from build123d import *

# Parameters (mm, degrees)
CROQUIS1_W              = 31.5
CROQUIS1_H              = 126
SALIENTE_EXTRUIR1_DEPTH = 4
CROQUIS3_R              = 2
CORTAR_EXTRUIR2_DEPTH   = 5
CROQUIS8_R              = 2.55
CORTAR_EXTRUIR3_DEPTH   = 5
CROQUIS11_R             = 1.575
CORTAR_EXTRUIR8_DEPTH   = 5
CROQUIS15_R             = 1.575
CORTAR_EXTRUIR11_DEPTH  = 5
CHAFL_N2_SIZE           = 3
CROQUIS19_R             = 3.5
CORTAR_EXTRUIR13_DEPTH  = 1.9
CROQUIS20_R             = 3.05
CORTAR_EXTRUIR14_DEPTH  = 2
CROQUIS24_W             = 31.5
CROQUIS24_H             = 3.76
SALIENTE_EXTRUIR3_DEPTH = 4
CROQUIS25_R             = 2.025
CORTAR_EXTRUIR15_DEPTH  = 5


with BuildPart() as part:
    # Croquis1 → Saliente-Extruir1 (new body)
    with BuildSketch(Plane(origin=(0, 0, 0), x_dir=(0, 0, -1), z_dir=(1, 0, 0))):
        Rectangle(CROQUIS1_W, CROQUIS1_H)
    extrude(amount=SALIENTE_EXTRUIR1_DEPTH)

    # Croquis3 → Cortar-Extruir2 (cut, through all)
    with BuildSketch(Plane(origin=(4, 0, 0), x_dir=(0, 0, -1), z_dir=(1, 0, 0))):
        with Locations((-10, 10.1)):
            Circle(CROQUIS3_R)
        with Locations((10, 10.1)):
            Circle(CROQUIS3_R)
        with Locations((-10, -9.9)):
            Circle(CROQUIS3_R)
        with Locations((10, -9.9)):
            Circle(CROQUIS3_R)
    extrude(amount=-CORTAR_EXTRUIR2_DEPTH, mode=Mode.SUBTRACT)

    # Croquis8 → Cortar-Extruir3 (cut, through all)
    with BuildSketch(Plane.ZY):
        with Locations((0, 45.75)):
            Circle(CROQUIS8_R)
    extrude(amount=-CORTAR_EXTRUIR3_DEPTH, mode=Mode.SUBTRACT)

    # Croquis11 → Cortar-Extruir8 (cut, through all)
    with BuildSketch(Plane(origin=(4, 0, 0), x_dir=(0, 0, -1), z_dir=(1, 0, 0))):
        with Locations((2.75, 34.75)):
            Circle(CROQUIS11_R)
        with Locations((2.75, 24.75)):
            Circle(CROQUIS11_R)
    extrude(amount=-CORTAR_EXTRUIR8_DEPTH, mode=Mode.SUBTRACT)

    # Croquis15 → Cortar-Extruir11 (cut, through all)
    with BuildSketch(Plane(origin=(4, 0, 0), x_dir=(0, 0, -1), z_dir=(1, 0, 0))):
        with Locations((-11.15, 57.45)):
            Circle(CROQUIS15_R)
        with Locations((11.15, 57.45)):
            Circle(CROQUIS15_R)
        with Locations((-11.15, 25.1)):
            Circle(CROQUIS15_R)
        with Locations((11.15, 25.1)):
            Circle(CROQUIS15_R)
    extrude(amount=-CORTAR_EXTRUIR11_DEPTH, mode=Mode.SUBTRACT)

    # Chaflán2
    chafl_n2_edges = [part.edges().sort_by_distance(p)[0] for p in [
        (2, 63, 15.75),
        (2, 63, -15.75),
    ]]
    chamfer(chafl_n2_edges, length=CHAFL_N2_SIZE)

    # Croquis19 → Cortar-Extruir13 (cut)
    with BuildSketch(Plane.ZY):
        with Locations((-2.75, 24.75)):
            Circle(CROQUIS19_R)
        with Locations((-2.75, 34.75)):
            Circle(CROQUIS19_R)
    extrude(amount=-CORTAR_EXTRUIR13_DEPTH, mode=Mode.SUBTRACT)

    # Croquis20 → Cortar-Extruir14 (cut)
    with BuildSketch(Plane(origin=(4, 0, 0), x_dir=(0, 0, -1), z_dir=(1, 0, 0))):
        with Locations((-11.15, 57.45)):
            Circle(CROQUIS20_R)
        with Locations((11.15, 57.45)):
            Circle(CROQUIS20_R)
        with Locations((11.15, 25.1)):
            Circle(CROQUIS20_R)
        with Locations((-11.15, 25.1)):
            Circle(CROQUIS20_R)
    extrude(amount=-CORTAR_EXTRUIR14_DEPTH, mode=Mode.SUBTRACT)

    # Croquis24 → Saliente-Extruir3 (add)
    with BuildSketch(Plane(origin=(4, 0, 0), x_dir=(0, 0, -1), z_dir=(1, 0, 0))):
        with Locations((0, -64.88)):
            Rectangle(CROQUIS24_W, CROQUIS24_H)
    extrude(amount=-SALIENTE_EXTRUIR3_DEPTH)

    # Croquis25 → Cortar-Extruir15 (cut, through all)
    with BuildSketch(Plane(origin=(4, 0, 0), x_dir=(0, 0, -1), z_dir=(1, 0, 0))):
        with Locations((-4.91726189, -23.891280092)):
            Circle(CROQUIS25_R)
        with Locations((-4.91726189, -33.891280092)):
            Circle(CROQUIS25_R)
    extrude(amount=-CORTAR_EXTRUIR15_DEPTH, mode=Mode.SUBTRACT)


solid = part.part
Source: CAD feature listing. Evaluate the final solid. Frame: model axes, mm. A direction names the side the tool comes from. Round coordinates to 2 decimals unless told otherwise and drop trailing zeros. Order: outer loops, then holes, each group sorted by start corner. A loop starts at its lowest first (then second) coordinate and runs counter-clockwise, first axis right, second up. Notation, with made-up numbers: (26, 22) - (52, 22) arc R11 ccw to (52, 42) - close; hole circle Ø5 at (-36, -14.75). An arc over 180 degrees is marked (long way). Use a Markdown table: item, result. Add a question column.
1. First-contact query: pin 1 (3.5 mm diameter, centred on y = 34.75, z = -2.75, fed in from -X); pin 2 (4 mm diameter, centred on y = 57.45, z = -11.15, fed in from +X). Flat tips, straight axial feed; report the tip coordinate or a pass-through.
2. Mould query, pull axis Y, two halves, no side actions, for faces 1 (the flat face through (2, 63, 0)), 2 (the cylindrical face through (2.965, 23.212, -2.409)), 3 (the flat face through (2, -4, -15.75)). Classes: +Y half, -Y half, draft (parallel to the pull), parting line (faces both ways), or undercut.
3. Section query C-C (x = 3). Give the number of separate pieces and of enclosed holes in the cut face, then the cut area to 3 significant figures.
4. Section query A-A (y = 34.75). Return the cut outline in (x, z) (3 decimals).
5. Section query B-B (y = -9.9). Return the cut outline in (x, z), then the cut area to 3 significant figures.
6. Set-up query: faces 4 (the flat face through (1.97, 61.48, -14.27)), 5 (the cylindrical face through (3.01, 27.67, -12.79)), 6 (the flat face through (1.9, 24, -1)). Return all of +Z, -Z, +X, -X, +Y, -Y with unobstructed straight access to the full face (end or side cutting, diameter ignored); none if empty.
7. Line query: probe 1 along Y at (x, z) = (0.3, 5); probe 2 along Y at (x, z) = (0.4, -4.5); probe 3 along Y at (x, z) = (1.7, -10). Output: solid intervals per line, ascending.
8. Section query D-D (z = 5). Return the cut outline in (x, y), then the cut area to 3 significant figures.
Derived:
| question | item | result |
|---|---|---|
| 1 | pin 1 | x = 1.9 |
| 1 | pin 2 | x = 2 |
| 2 | face 1 | +Y half |
| 2 | face 2 | undercut |
| 2 | face 3 | draft |
| 3 | separate pieces | 1 |
| 3 | enclosed holes | 13 |
| 3 | area | 3,850 mm2 |
| 4 | outline | (0, -15.75) - (4, -15.75) - (4, -4.325) - (1.9, -4.325) - (1.9, -6.25) - (0, -6.25) - close; (0, 0.75) - (1.9, 0.75) - (1.9, -1.175) - (4, -1.175) - (4, 15.75) - (0, 15.75) - close |
| 5 | outline | (0, -15.75) - (4, -15.75) - (4, -12) - (0, -12) - close; (0, -8) - (4, -8) - (4, 8) - (0, 8) - close; (0, 12) - (4, 12) - (4, 15.75) - (0, 15.75) - close |
| 5 | area | 94.0 mm2 |
| 6 | face 4 | -Z, +X, -X, +Y |
| 6 | face 5 | +X |
| 6 | face 6 | -X |
| 7 | probe 1 | -66.76 to -35.91, -31.87 to -25.91, -21.87 to 63 |
| 7 | probe 2 | -66.76 to 21.72, 27.78 to 31.72, 37.78 to 63 |
| 7 | probe 3 | -66.76 to -11.9, -7.9 to 8.1, 12.1 to 24.02, 26.18 to 56.37, 58.53 to 63 |
| 8 | outline | (0, -66.76) - (4, -66.76) - (4, -35.91) - (0, -35.91) - close; (0, -31.87) - (4, -31.87) - (4, -25.91) - (0, -25.91) - close; (0, -21.87) - (4, -21.87) - (4, 63) - (0, 63) - close |
| 8 | area | 487 mm2 |
